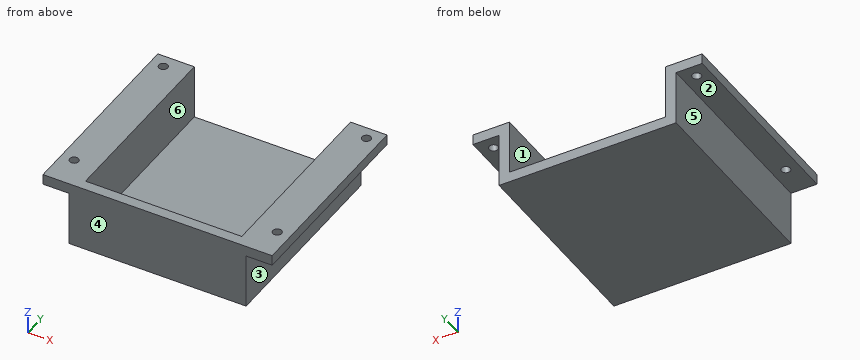
```python
from build123d import *

# Parameters (mm, degrees)
BOSS_EXTRUDE1_DEPTH = 76
SKETCH2_W           = 60
SKETCH2_H           = 4
EXTRUDE_THIN1_DEPTH = 21
SKETCH4_R           = 1.7
CUT_EXTRUDE1_DEPTH  = 21


with BuildPart() as part:
    # Sketch1 → Boss-Extrude1 (new body)
    with BuildSketch(Plane(origin=(0, 0, 0), x_dir=(1, 0, 0), z_dir=(0, 1, 0))):
        Polygon((-48.166666667, 0), (-38.166666667, 0), (-38.166666667, 21), (29.833333333, 21), (29.833333333, 0), (39.833333333, 0), (39.833333333, -4), (25.833333333, -4), (25.833333333, 17), (-34.166666667, 17), (-34.166666667, -4), (-48.166666667, -4), align=None)
    extrude(amount=BOSS_EXTRUDE1_DEPTH)

    # Sketch2 → Extrude-Thin1 (add)
    with BuildSketch(Plane.XY.offset(-17)):
        with Locations((-4.166666667, 2)):
            Rectangle(SKETCH2_W, SKETCH2_H)
    extrude(amount=EXTRUDE_THIN1_DEPTH)

    # Sketch4 → Cut-Extrude1 (cut)
    with BuildSketch(Plane(origin=(0, 0, 0), x_dir=(-1, 0, 0), z_dir=(0, 0, -1))):
        with Locations((-34.833333333, 71)):
            Circle(SKETCH4_R)
        with Locations((-34.833333333, 12)):
            Circle(SKETCH4_R)
        with Locations((43.166666667, 71)):
            Circle(SKETCH4_R)
        with Locations((43.166666667, 12)):
            Circle(SKETCH4_R)
    extrude(amount=-CUT_EXTRUDE1_DEPTH, mode=Mode.SUBTRACT)


solid = part.part
```
Can you work these out from the model? Positions are in its coordinate system, mm. Face numbers are marked on the shaded views. A direction names the side the tool comes from. Coordinates: 2 decimals unless noted, no trailing zeros. Loops run counter-clockwise (first coordinate to the right, second up) from the corner with the lowest first, then second, coordinate; pieces in that order, holes last.
1) Imagine slicing it at B-B on z = -11. List the corners of the cut face in (x, y) for me, plus the area to 3 significant figures.
2) For pin 1 (6.5 mm diameter, centred on y = 31, z = -12, fed in from -X); pin 2 (3 mm diameter, centred on x = -42, y = 50.5, fed in from -Z); pin 3 (3 mm diameter, centred on y = 54.5, z = -12, fed in from +X), each with a flat end and sliding along its axis, tell me the tip position at first contact or that it passes through.
3) Imagine slicing it at A-A on y = 12. List the corners of the cut face in (x, z) for me.
4) Thinking about a two-plate mould opening in X: for the marked faces 4, 5 and 6, which applies, pulls with the +X half, pulls with the -X half, needs draft (parallel to the pull), parting line crosses it, or undercut?
5) Which directions (+Z, -Z, +X, -X, +Y, -Y) give clear straight access to the entire face, cutting with the end or side of a thin tool? Please do the marked faces 1, 2 and 3.
6) Imagine slicing it at C-C on z = 1.25. List the corners of the cut face in (x, y) for me, plus the area to 3 significant figures.
7) Imagine slicing it at D-D on x = 20. List the corners of the cut face in (y, z) for me.
8) I need wall thicknesses on probe 1 along X at (y, z) = (71, 3.05); probe 2 along X at (y, z) = (56, -6); probe 3 along Z at (x, y) = (-27.5, 10). Which ranges of each line are inside material? Lowest first, please.
Completed:
1. outline: (-38.17, 0) - (29.83, 0) - (29.83, 76) - (25.83, 76) - (25.83, 4) - (-34.17, 4) - (-34.17, 76) - (-38.17, 76) - close
1. area: 848 mm2
2. pin 1: stops at x = -38.17
2. pin 2: stops at z = 0
2. pin 3: stops at x = 29.83
3. outline: (-48.17, 0) - (-44.87, 0) - (-44.87, 4) - (-48.17, 4) - close; (-41.47, 0) - (-38.17, 0) - (-38.17, -21) - (29.83, -21) - (29.83, 0) - (33.13, 0) - (33.13, 4) - (25.83, 4) - (25.83, -17) - (-34.17, -17) - (-34.17, 4) - (-41.47, 4) - close; (36.53, 0) - (39.83, 0) - (39.83, 4) - (36.53, 4) - close
4. face 4: needs draft
4. face 5: pulls with the -X half
4. face 6: undercut
5. face 1: +Z, +Y
5. face 2: -Z, -X, +Y, -Y
5. face 3: -Z, +X, +Y, -Y
6. outline: (-48.17, 0) - (39.83, 0) - (39.83, 76) - (25.83, 76) - (25.83, 4) - (-34.17, 4) - (-34.17, 76) - (-48.17, 76) - close; hole circle Ø3.4 at (-43.17, 12); hole circle Ø3.4 at (-43.17, 71); hole circle Ø3.4 at (34.83, 12); hole circle Ø3.4 at (34.83, 71)
6. area: 2,330 mm2
7. outline: (0, -21) - (76, -21) - (76, -17) - (4, -17) - (4, 4) - (0, 4) - close
8. probe 1: x = -48.17 to -44.87, -41.47 to -34.17, 25.83 to 33.13, 36.53 to 39.83
8. probe 2: x = -38.17 to -34.17, 25.83 to 29.83
8. probe 3: z = -21 to -17
